Geometry check sheet. Reference: the model listing, model coordinates, mm. Face numbers are marked on the shaded views. Round coordinates to 2 decimals unless told otherwise and drop trailing zeros. Use a Markdown table: item, result.
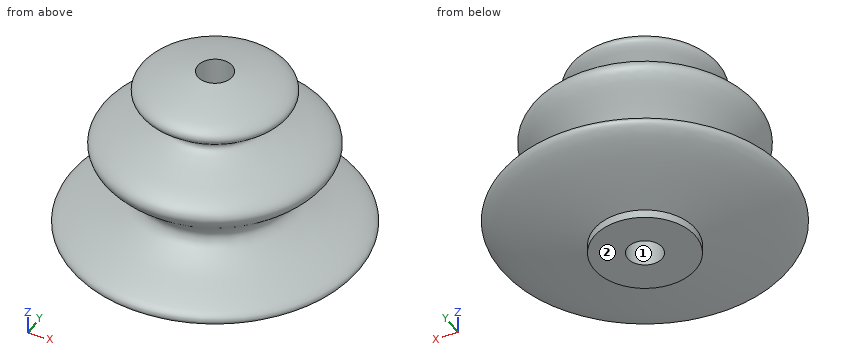
```python
from build123d import *

# Parameters (mm, degrees)
F2_R     = 9.3394662064
F3_DEPTH = 12.7
F5_D     = 6.35


with BuildPart() as f1:
    # F0 (on Front) → F1 (revolve)
    with BuildSketch(Plane.XZ):
        with BuildLine():
            Line((0, 38.1), (0, 0))
            add(Edge.make_bspline(
                [(0, 0), (14.350977372, 2.2945801413), (39.1855557702, 6.2653849814), (4.3012712165, 12.7381315434), (29.7354424134, 24.2806495401), (2.422248214, 27.9041384292), (19.3085066306, 34.3315694195), (7.2616463998, 36.6827484807), (0, 38.1)],
                knots=[0, 0, 0, 0, 0.2339384907, 0.4048340149, 0.5558357804, 0.7180755229, 0.8300606279, 1, 1, 1, 1], degree=3))
        make_face()
    revolve(axis=Axis((0, 0, 19.05), (0, 0, -1)))

    # F2 (on Top) → F3 (join)
    with BuildSketch(Plane.XY):
        Circle(F2_R)
    extrude(amount=F3_DEPTH)

    # F5 (through all)
    with Locations(Plane(origin=(0, 0, 0), x_dir=(1, 0, 0), z_dir=(0, 0, -1))):
        with Locations((0, 0)):
            Hole(F5_D / 2)


solid = f1.part
```
(1) Thickness scan on line 1 (X direction, y = -2, z = 14); line 2 (Z direction, x = -9, y = -13); line 3 (Z direction, x = 14, y = -7.5). Record the ranges inside material, lowest first.
A:
| item | result |
|---|---|
| line 1 | x = -13.37 to -2.47, 2.47 to 13.37 |
| line 2 | z = 2.7 to 11.69, 17.41 to 25.83 |
| line 3 | z = 2.72 to 11.65, 17.47 to 25.81 |
(2) Release check for a two-part mould opening along Y. For the marked faces 1 and 2 record: +Y half, -Y half, draft (parallel to the pull), parting line (faces both ways), or undercut.
A:
| item | result |
|---|---|
| face 1 | undercut |
| face 2 | draft |
(3) Gauge pin test, flat ends, axial feed: pin 1 Ø5.5 at (x, y) = (0, 0) entering from +Z; pin 2 Ø1 at (x, z) = (1, 23.5) entering from -Y; pin 3 Ø3 at (x, y) = (4.5, -17) entering from -Z; pin 4 Ø1.5 at (x, z) = (0, 15) entering from -Y. Record the tip position at first contact, or that the pin passes through.
A:
| item | result |
|---|---|
| pin 1 | passes through |
| pin 2 | stops at y = -20.59 |
| pin 3 | stops at z = 2.76 |
| pin 4 | stops at y = -14.18 |
